from build123d import *

# Parameters (mm, degrees)
F0_W     = 70
F0_H     = 34
F1_DEPTH = 12
F2_DEPTH = 7
F3_R     = 4
F4_DEPTH = 34.001
F5_R     = 5


# Not quite as in the source:
# - a feature names something its author has since deleted; it is built from what else it names


with BuildPart() as f1:
    # F0 (on Top) → F1 (new body)
    with BuildSketch(Plane.XY):
        Rectangle(F0_W, F0_H)
        with BuildLine():
            Line((-6, -15.1), (-18, -15.1))
            ThreePointArc((-18, -15.1), (-23.1, -10), (-18, -4.9))
            Line((-18, -4.9), (-6, -4.9))
            ThreePointArc((-6, -4.9), (-0.9, -10), (-6, -15.1))
        make_face(mode=Mode.SUBTRACT)
        with BuildLine():
            ThreePointArc((6, -15.1), (0.9, -10), (6, -4.9))
            Line((6, -4.9), (18, -4.9))
            ThreePointArc((18, -4.9), (23.1, -10), (18, -15.1))
            Line((18, -15.1), (6, -15.1))
        make_face(mode=Mode.SUBTRACT)
        with BuildLine():
            Line((-18, 15.1), (-6, 15.1))
            ThreePointArc((-6, 15.1), (-0.9, 10), (-6, 4.9))
            Line((-6, 4.9), (-18, 4.9))
            ThreePointArc((-18, 4.9), (-23.1, 10), (-18, 15.1))
        make_face(mode=Mode.SUBTRACT)
        with BuildLine():
            ThreePointArc((6, 4.9), (0.9, 10), (6, 15.1))
            Line((6, 15.1), (18, 15.1))
            ThreePointArc((18, 15.1), (23.1, 10), (18, 4.9))
            Line((18, 4.9), (6, 4.9))
        make_face(mode=Mode.SUBTRACT)
    extrude(amount=F1_DEPTH)

    # F0 (on Top) → F2 (join)
    with BuildSketch(Plane.XY):
        with BuildLine():
            ThreePointArc((-6, 4.9), (-0.9, 10), (-6, 15.1))
            Line((-6, 15.1), (-18, 15.1))
            ThreePointArc((-18, 15.1), (-23.1, 10), (-18, 4.9))
            Line((-18, 4.9), (-6, 4.9))
        make_face()
        with BuildLine():
            Line((-18, 12.6), (-6, 12.6))
            ThreePointArc((-6, 12.6), (-3.4, 10), (-6, 7.4))
            Line((-6, 7.4), (-18, 7.4))
            ThreePointArc((-18, 7.4), (-20.6, 10), (-18, 12.6))
        make_face(mode=Mode.SUBTRACT)
        with BuildLine():
            Line((18, 15.1), (6, 15.1))
            ThreePointArc((6, 15.1), (0.9, 10), (6, 4.9))
            Line((6, 4.9), (18, 4.9))
            ThreePointArc((18, 4.9), (23.1, 10), (18, 15.1))
        make_face()
        with BuildLine():
            ThreePointArc((6, 7.4), (3.4, 10), (6, 12.6))
            Line((6, 12.6), (18, 12.6))
            ThreePointArc((18, 12.6), (20.6, 10), (18, 7.4))
            Line((18, 7.4), (6, 7.4))
        make_face(mode=Mode.SUBTRACT)
        with BuildLine():
            Line((18, -4.9), (6, -4.9))
            ThreePointArc((6, -4.9), (0.9, -10), (6, -15.1))
            Line((6, -15.1), (18, -15.1))
            ThreePointArc((18, -15.1), (23.1, -10), (18, -4.9))
        make_face()
        with BuildLine():
            Line((18, -12.6), (6, -12.6))
            ThreePointArc((6, -12.6), (3.4, -10), (6, -7.4))
            Line((6, -7.4), (18, -7.4))
            ThreePointArc((18, -7.4), (20.6, -10), (18, -12.6))
        make_face(mode=Mode.SUBTRACT)
        with BuildLine():
            ThreePointArc((-18, -4.9), (-23.1, -10), (-18, -15.1))
            Line((-18, -15.1), (-6, -15.1))
            ThreePointArc((-6, -15.1), (-0.9, -10), (-6, -4.9))
            Line((-6, -4.9), (-18, -4.9))
        make_face()
        with BuildLine():
            Line((-6, -12.6), (-18, -12.6))
            ThreePointArc((-18, -12.6), (-20.6, -10), (-18, -7.4))
            Line((-18, -7.4), (-6, -7.4))
            ThreePointArc((-6, -7.4), (-3.4, -10), (-6, -12.6))
        make_face(mode=Mode.SUBTRACT)
    extrude(amount=F2_DEPTH)

    # F3 (on face) → F4 (cut, through all)
    with BuildSketch(Plane(origin=(0, 17, 0), x_dir=(-1, 0, 0), z_dir=(0, 1, 0))):
        with Locations((28, 6)):
            Circle(F3_R)
        with Locations((-28, 6)):
            Circle(F3_R)
    extrude(amount=-F4_DEPTH, mode=Mode.SUBTRACT)

    # F5
    f5_edges = [f1.edges().sort_by_distance(p)[0] for p in [
        (-35, 0, 12),
        (35, 0, 12),
        (-35, 0, 0),
        (35, 0, 0),
    ]]
    fillet(f5_edges, radius=F5_R)


solid = f1.part
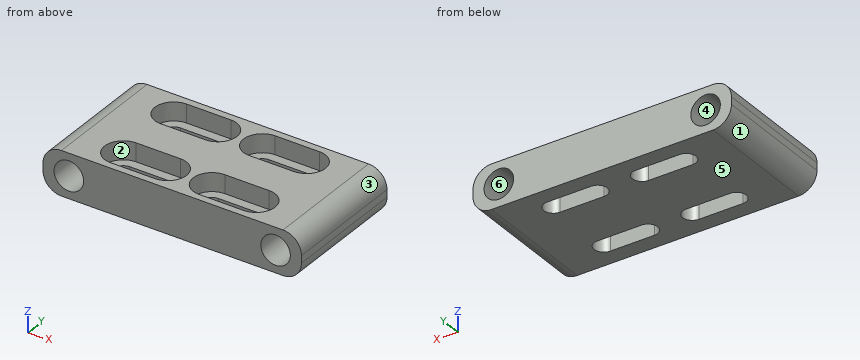
Design review of the part built by this model. Coordinates are the model's own, in mm. Face numbers are marked on the shaded views. A direction names the side the tool comes from. Round coordinates to 2 decimals unless told otherwise and drop trailing zeros. Loops run counter-clockwise (first coordinate to the right, second up) from the corner with the lowest first, then second, coordinate; pieces in that order, holes last. Notation, with made-up numbers: M -2.75,-12 L 35.25,-12 A28 ccw 35.25,24 Z; hole C -31,-31.5 d1. An arc over 180 degrees is marked long. Answer as a JSON object with one key per item and string values.
Item 1: We need section C-C on x = 14. Give the boundary of the cut face in (y, z), and give its area (3 significant figures).
Answer sheet:
{"outline": "M -17,0 L -12.6,0 L -12.6,7 L -15.1,7 L -15.1,12 L -17,12 Z; M -7.4,0 L 7.4,0 L 7.4,7 L 4.9,7 L 4.9,12 L -4.9,12 L -4.9,7 L -7.4,7 Z; M 12.6,0 L 17,0 L 17,12 L 15.1,12 L 15.1,7 L 12.6,7 Z", "area": "233 mm^2"}
Item 2: We need section D-D on y = 3. Give the boundary of the cut face in (x, z).
Answer sheet:
{"outline": "M -35,5 A5 ccw -30,0 L 30,0 A5 ccw 35,5 L 35,7 A5 ccw 30,12 L -30,12 A5 ccw -35,7 Z; hole C -28,6 d8; hole C 28,6 d8"}
Item 3: Wall thickness on L1, parallel to Y at x = 8, z = 9.75; L2, parallel to Y at x = 17, z = 3.25; L3, parallel to X at y = 9, z = 6.25: over which ranges is each line inside the solid? List them lowest first. Write a range as from..to.
Answer sheet:
{"L1": "y = -17..-15.1, -4.9..4.9, 15.1..17", "L2": "y = -17..-12.6, -7.4..7.4, 12.6..17", "L3": "x = -35..-31.99, -24.01..-20.4, -3.6..3.6, 20.4..24.01, 31.99..35"}
Item 4: Clearance check with a flat-ended pin moving along its axis: P1, Ø8, axis at x = -8.5, y = 9, coming from the +Z side. State where the tip first meets the part, or that it passes through.
Answer sheet:
{"P1": "stops at z = 7"}
Item 5: The part is to be moulded in two halves that separate along X. For the marked faces 3, 4, 5 and 6, say which applies: pulls with the +X half, pulls with the -X half, needs draft (parallel to the pull), parting line crosses it, or undercut.
Answer sheet:
{"face 3": "pulls with the +X half", "face 4": "undercut", "face 5": "needs draft", "face 6": "undercut"}
Item 6: We need section B-B on z = 6. Give the boundary of the cut face in (x, y), and give its area (3 significant figures).
Answer sheet:
{"outline": "M -35,-17 L -32,-17 L -32,17 L -35,17 Z; M -24,-17 L 24,-17 L 24,17 L -24,17 Z; M 32,-17 L 35,-17 L 35,17 L 32,17 Z; hole M -18,-12.6 L -6,-12.6 A2.6 ccw -6,-7.4 L -18,-7.4 A2.6 ccw Z; hole M -18,7.4 L -6,7.4 A2.6 ccw -6,12.6 L -18,12.6 A2.6 ccw Z; hole M 6,-12.6 L 18,-12.6 A2.6 ccw 18,-7.4 L 6,-7.4 A2.6 ccw Z; hole M 6,7.4 L 18,7.4 A2.6 ccw 18,12.6 L 6,12.6 A2.6 ccw Z", "area": "1,500 mm^2"}
Item 7: We need section A-A on y = 10. Give the boundary of the cut face in (x, z).
Answer sheet:
{"outline": "M -35,5 A5 ccw -30,0 L -20.6,0 L -20.6,7 L -23.1,7 L -23.1,12 L -30,12 A5 ccw -35,7 Z; M -3.4,0 L 3.4,0 L 3.4,7 L 0.9,7 L 0.9,12 L -0.9,12 L -0.9,7 L -3.4,7 Z; M 20.6,0 L 30,0 A5 ccw 35,5 L 35,7 A5 ccw 30,12 L 23.1,12 L 23.1,7 L 20.6,7 Z; hole C -28,6 d8; hole C 28,6 d8"}
Item 8: Machinability: for the marked faces 1 and 2, which of the approach directions +Z, -Z, +X, -X, +Y, -Y give a long, thin tool a straight path to every point of the face, cutting with its end or side? Answer none if there is none.
Answer sheet:
{"face 1": "-Z, -X, +Y, -Y", "face 2": "+Z"}
